Source: three-view drawing plus pictorial views. Frame: mm from the lowest corner of the part. A direction names the side the tool comes from. Round coordinates to 2 decimals unless told otherwise and drop trailing zeros. Loops run counter-clockwise (first coordinate to the right, second up) from the corner with the lowest first, then second, coordinate; pieces in that order, holes last. Notation, with made-up numbers: (14, 44) -> (26, 44) arc R12 ccw to (26, 67) -> close; hole circle Ø6 at (28.5, 47). An arc over 180 degrees is marked (long way). One line per question, with ' | ' between items. Start each with the question number.
Q1. Cut plane B-B on z = 7. Return loops of the section in (x, y).
Q2. Cut plane C-C on x = 37. Return loops of the section in (y, z).
Q3. Contact query for flat-ended pins moving along their axis: P1, Ø6, axis at y = 9.5, z = 5.5, coming from the +X side; P2, Ø4, axis at y = 24, z = 7, coming from the -X side; P3, Ø3.5, axis at x = 38.5, z = 10, coming from the +Y side. Output: stop coordinate, or through.
Q4. Cut plane A-A on y = 20. Return loops of the section in (x, z), and give its area (3 significant figures).
Q5. Access query for the marked faces 1, 2 and 3. Directions: +Z, -Z, +X, -X, +Y, -Y. A direction counts if a zero-diameter tool reaches every point of the face in a straight line with its end or side. Return the directions, or none.
Q6. Cut plane D-D on z = 12. Return loops of the section in (x, y).
Q7. Mould query, pull axis X, two halves, no side actions, for the marked faces 4, 5 and 6. Classes: pulls with the +X half, pulls with the -X half, needs draft (parallel to the pull), parting line crosses it, or undercut.
Q8. Material intervals for L1, parallel to X at y = 1.45, z = 7; L2, parallel to X at y = 20, z = 9.5; L3, parallel to X at y = 29.5, z = 7.5, sorted ascending.
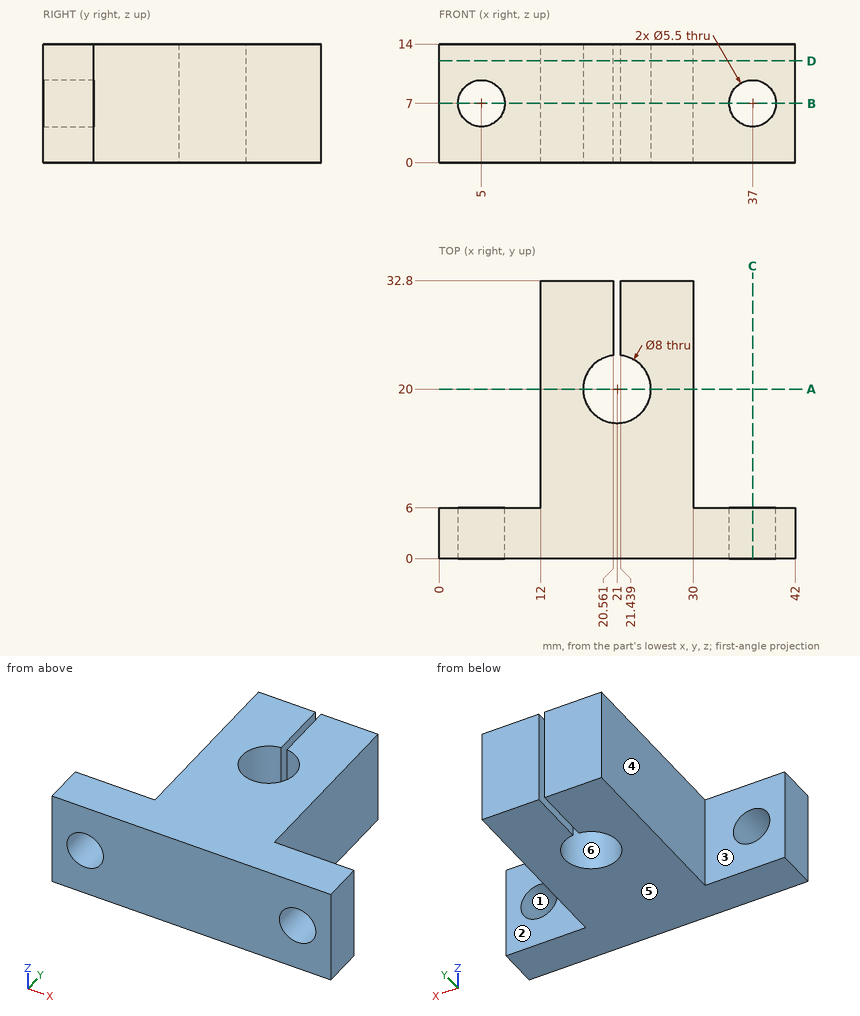
Results:
1) outline: (0, 0) -> (2.25, 0) -> (2.25, 6) -> (0, 6) -> close; (7.75, 0) -> (34.25, 0) -> (34.25, 6) -> (30, 6) -> (30, 32.8) -> (21.44, 32.8) -> (21.44, 23.98) arc R4 cw (long way) to (20.56, 23.98) -> (20.56, 32.8) -> (12, 32.8) -> (12, 6) -> (7.75, 6) -> close; (39.75, 0) -> (42, 0) -> (42, 6) -> (39.75, 6) -> close
2) outline: (0, 0) -> (6, 0) -> (6, 4.25) -> (0, 4.25) -> close; (0, 9.75) -> (6, 9.75) -> (6, 14) -> (0, 14) -> close
3) P1: x = 30 | P2: x = 12 | P3: y = 6
4) outline: (12, 0) -> (17, 0) -> (17, 14) -> (12, 14) -> close; (25, 0) -> (30, 0) -> (30, 14) -> (25, 14) -> close | area: 140 mm^2
5) face 1: +Y, -Y | face 2: +Z, -Z, +X, +Y | face 3: +Z, -Z, -X, +Y
6) outline: (0, 0) -> (42, 0) -> (42, 6) -> (30, 6) -> (30, 32.8) -> (21.44, 32.8) -> (21.44, 23.98) arc R4 cw (long way) to (20.56, 23.98) -> (20.56, 32.8) -> (12, 32.8) -> (12, 6) -> (0, 6) -> close
7) face 4: pulls with the -X half | face 5: needs draft | face 6: undercut
8) L1: 0 to 2.25, 7.75 to 34.25, 39.75 to 42 | L2: 12 to 17, 25 to 30 | L3: 12 to 20.56, 21.44 to 30
